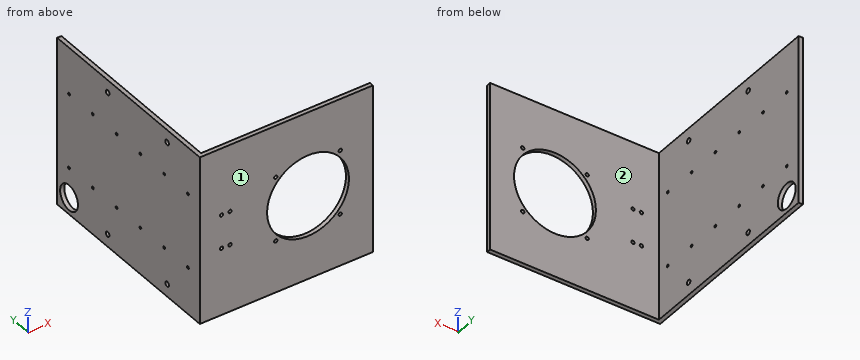
from build123d import *

# Parameters (mm, degrees)
BOSS_EXTRUDE1_DEPTH = 200
CUT_EXTRUDE1_REACH  = 372.473
SKETCH2_R           = 48.5
SKETCH2_R_2         = 2
CUT_EXTRUDE2_REACH  = 372.473
SKETCH3_R           = 2
SKETCH4_R           = 15
CUT_EXTRUDE3_DEPTH  = 10
CUT_EXTRUDE4_REACH  = 372.945
SKETCH5_R           = 3
CUT_EXTRUDE5_REACH  = 372.945
SKETCH6_R           = 1.5


with BuildPart() as part:
    # Sketch1 → Boss-Extrude1 (new body)
    with BuildSketch(Plane.XY):
        Polygon((0, 240), (0, 0), (205, 0), (205, 5), (5, 5), (5, 240), align=None)
    extrude(amount=BOSS_EXTRUDE1_DEPTH)

    # Sketch2 → Cut-Extrude1 (cut, up to next)
    with BuildSketch(Plane(origin=(0, 5, 0), x_dir=(1, 0, 0), z_dir=(0, 1, 0)), mode=Mode.PRIVATE) as cut_extrude1_sk1:
        with Locations(Location((128.16761425, -100, 0), (0, 0, 180))):
            Circle(SKETCH2_R)
    cut_extrude1_tool1 = extrude(cut_extrude1_sk1.sketch, amount=-CUT_EXTRUDE1_REACH, mode=Mode.PRIVATE) & part.part
    # Sketch2 → Cut-Extrude1 (cut, up to next)
    with BuildSketch(Plane(origin=(0, 5, 0), x_dir=(1, 0, 0), z_dir=(0, 1, 0)), mode=Mode.PRIVATE) as cut_extrude1_sk2:
        with Locations(Location((89.98261425, -61.817467672, 0), (0, 0, 180))):
            Circle(SKETCH2_R_2)
    cut_extrude1_tool2 = extrude(cut_extrude1_sk2.sketch, amount=-CUT_EXTRUDE1_REACH, mode=Mode.PRIVATE) & part.part
    # Sketch2 → Cut-Extrude1 (cut, up to next)
    with BuildSketch(Plane(origin=(0, 5, 0), x_dir=(1, 0, 0), z_dir=(0, 1, 0)), mode=Mode.PRIVATE) as cut_extrude1_sk3:
        with Locations(Location((166.35261425, -61.817467672, 0), (0, 0, 180))):
            Circle(SKETCH2_R_2)
    cut_extrude1_tool3 = extrude(cut_extrude1_sk3.sketch, amount=-CUT_EXTRUDE1_REACH, mode=Mode.PRIVATE) & part.part
    # Sketch2 → Cut-Extrude1 (cut, up to next)
    with BuildSketch(Plane(origin=(0, 5, 0), x_dir=(1, 0, 0), z_dir=(0, 1, 0)), mode=Mode.PRIVATE) as cut_extrude1_sk4:
        with Locations(Location((89.98261425, -138.182532328, 0), (0, 0, 180))):
            Circle(SKETCH2_R_2)
    cut_extrude1_tool4 = extrude(cut_extrude1_sk4.sketch, amount=-CUT_EXTRUDE1_REACH, mode=Mode.PRIVATE) & part.part
    # Sketch2 → Cut-Extrude1 (cut, up to next)
    with BuildSketch(Plane(origin=(0, 5, 0), x_dir=(1, 0, 0), z_dir=(0, 1, 0)), mode=Mode.PRIVATE) as cut_extrude1_sk5:
        with Locations(Location((166.35261425, -138.182532328, 0), (0, 0, 180))):
            Circle(SKETCH2_R_2)
    cut_extrude1_tool5 = extrude(cut_extrude1_sk5.sketch, amount=-CUT_EXTRUDE1_REACH, mode=Mode.PRIVATE) & part.part
    add(cut_extrude1_tool1.solids().sort_by_distance((128.167614, 5, 100))[0], mode=Mode.SUBTRACT)
    add(cut_extrude1_tool2.solids().sort_by_distance((89.982614, 5, 61.817468))[0], mode=Mode.SUBTRACT)
    add(cut_extrude1_tool3.solids().sort_by_distance((166.352614, 5, 61.817468))[0], mode=Mode.SUBTRACT)
    add(cut_extrude1_tool4.solids().sort_by_distance((89.982614, 5, 138.182532))[0], mode=Mode.SUBTRACT)
    add(cut_extrude1_tool5.solids().sort_by_distance((166.352614, 5, 138.182532))[0], mode=Mode.SUBTRACT)

    # Sketch3 → Cut-Extrude2 (cut, up to next)
    with BuildSketch(Plane(origin=(0, 5, 0), x_dir=(1, 0, 0), z_dir=(0, 1, 0)), mode=Mode.PRIVATE) as cut_extrude2_sk1:
        with Locations(Location((25.75, -80, 0), (0, 0, 180))):
            Circle(SKETCH3_R)
    cut_extrude2_tool1 = extrude(cut_extrude2_sk1.sketch, amount=-CUT_EXTRUDE2_REACH, mode=Mode.PRIVATE) & part.part
    # Sketch3 → Cut-Extrude2 (cut, up to next)
    with BuildSketch(Plane(origin=(0, 5, 0), x_dir=(1, 0, 0), z_dir=(0, 1, 0)), mode=Mode.PRIVATE) as cut_extrude2_sk2:
        with Locations(Location((25.75, -120, 0), (0, 0, 270))):
            Circle(SKETCH3_R)
    cut_extrude2_tool2 = extrude(cut_extrude2_sk2.sketch, amount=-CUT_EXTRUDE2_REACH, mode=Mode.PRIVATE) & part.part
    # Sketch3 → Cut-Extrude2 (cut, up to next)
    with BuildSketch(Plane(origin=(0, 5, 0), x_dir=(1, 0, 0), z_dir=(0, 1, 0)), mode=Mode.PRIVATE) as cut_extrude2_sk3:
        with Locations(Location((35.75, -120, 0), (0, 0, 180))):
            Circle(SKETCH3_R)
    cut_extrude2_tool3 = extrude(cut_extrude2_sk3.sketch, amount=-CUT_EXTRUDE2_REACH, mode=Mode.PRIVATE) & part.part
    # Sketch3 → Cut-Extrude2 (cut, up to next)
    with BuildSketch(Plane(origin=(0, 5, 0), x_dir=(1, 0, 0), z_dir=(0, 1, 0)), mode=Mode.PRIVATE) as cut_extrude2_sk4:
        with Locations(Location((35.75, -80, 0), (0, 0, 270))):
            Circle(SKETCH3_R)
    cut_extrude2_tool4 = extrude(cut_extrude2_sk4.sketch, amount=-CUT_EXTRUDE2_REACH, mode=Mode.PRIVATE) & part.part
    add(cut_extrude2_tool1.solids().sort_by_distance((25.75, 5, 80))[0], mode=Mode.SUBTRACT)
    add(cut_extrude2_tool2.solids().sort_by_distance((25.75, 5, 120))[0], mode=Mode.SUBTRACT)
    add(cut_extrude2_tool3.solids().sort_by_distance((35.75, 5, 120))[0], mode=Mode.SUBTRACT)
    add(cut_extrude2_tool4.solids().sort_by_distance((35.75, 5, 80))[0], mode=Mode.SUBTRACT)

    # Sketch4 → Cut-Extrude3 (cut)
    with BuildSketch(Plane(origin=(5, 0, 0), x_dir=(0, 0, -1), z_dir=(1, 0, 0))):
        with Locations(Location((-20, 220, 0), (0, 0, 90))):
            Circle(SKETCH4_R)
    extrude(amount=-CUT_EXTRUDE3_DEPTH, mode=Mode.SUBTRACT)

    # Sketch5 → Cut-Extrude4 (cut, up to next)
    with BuildSketch(Plane(origin=(5, 0, 0), x_dir=(0, 0, -1), z_dir=(1, 0, 0)), mode=Mode.PRIVATE) as cut_extrude4_sk1:
        with Locations(Location((-185, 55, 0), (0, 0, 90))):
            Circle(SKETCH5_R)
    cut_extrude4_tool1 = extrude(cut_extrude4_sk1.sketch, amount=-CUT_EXTRUDE4_REACH, mode=Mode.PRIVATE) & part.part
    # Sketch5 → Cut-Extrude4 (cut, up to next)
    with BuildSketch(Plane(origin=(5, 0, 0), x_dir=(0, 0, -1), z_dir=(1, 0, 0)), mode=Mode.PRIVATE) as cut_extrude4_sk2:
        with Locations(Location((-185, 155, 0), (0, 0, 90))):
            Circle(SKETCH5_R)
    cut_extrude4_tool2 = extrude(cut_extrude4_sk2.sketch, amount=-CUT_EXTRUDE4_REACH, mode=Mode.PRIVATE) & part.part
    # Sketch5 → Cut-Extrude4 (cut, up to next)
    with BuildSketch(Plane(origin=(5, 0, 0), x_dir=(0, 0, -1), z_dir=(1, 0, 0)), mode=Mode.PRIVATE) as cut_extrude4_sk3:
        with Locations(Location((-15, 55, 0), (0, 0, 90))):
            Circle(SKETCH5_R)
    cut_extrude4_tool3 = extrude(cut_extrude4_sk3.sketch, amount=-CUT_EXTRUDE4_REACH, mode=Mode.PRIVATE) & part.part
    # Sketch5 → Cut-Extrude4 (cut, up to next)
    with BuildSketch(Plane(origin=(5, 0, 0), x_dir=(0, 0, -1), z_dir=(1, 0, 0)), mode=Mode.PRIVATE) as cut_extrude4_sk4:
        with Locations(Location((-15, 155, 0), (0, 0, 90))):
            Circle(SKETCH5_R)
    cut_extrude4_tool4 = extrude(cut_extrude4_sk4.sketch, amount=-CUT_EXTRUDE4_REACH, mode=Mode.PRIVATE) & part.part
    add(cut_extrude4_tool1.solids().sort_by_distance((5, 55, 185))[0], mode=Mode.SUBTRACT)
    add(cut_extrude4_tool2.solids().sort_by_distance((5, 155, 185))[0], mode=Mode.SUBTRACT)
    add(cut_extrude4_tool3.solids().sort_by_distance((5, 55, 15))[0], mode=Mode.SUBTRACT)
    add(cut_extrude4_tool4.solids().sort_by_distance((5, 155, 15))[0], mode=Mode.SUBTRACT)

    # Sketch6 → Cut-Extrude5 (cut, up to next)
    with BuildSketch(Plane(origin=(5, 0, 0), x_dir=(0, 0, -1), z_dir=(1, 0, 0)), mode=Mode.PRIVATE) as cut_extrude5_sk1:
        with Locations(Location((-144.25, 220, 0), (0, 0, 90))):
            Circle(SKETCH6_R)
    cut_extrude5_tool1 = extrude(cut_extrude5_sk1.sketch, amount=-CUT_EXTRUDE5_REACH, mode=Mode.PRIVATE) & part.part
    # Sketch6 → Cut-Extrude5 (cut, up to next)
    with BuildSketch(Plane(origin=(5, 0, 0), x_dir=(0, 0, -1), z_dir=(1, 0, 0)), mode=Mode.PRIVATE) as cut_extrude5_sk2:
        with Locations(Location((-55.75, 220, 0), (0, 0, 90))):
            Circle(SKETCH6_R)
    cut_extrude5_tool2 = extrude(cut_extrude5_sk2.sketch, amount=-CUT_EXTRUDE5_REACH, mode=Mode.PRIVATE) & part.part
    # Sketch6 → Cut-Extrude5 (cut, up to next)
    with BuildSketch(Plane(origin=(5, 0, 0), x_dir=(0, 0, -1), z_dir=(1, 0, 0)), mode=Mode.PRIVATE) as cut_extrude5_sk3:
        with Locations(Location((-144.25, 180, 0), (0, 0, 90))):
            Circle(SKETCH6_R)
    cut_extrude5_tool3 = extrude(cut_extrude5_sk3.sketch, amount=-CUT_EXTRUDE5_REACH, mode=Mode.PRIVATE) & part.part
    # Sketch6 → Cut-Extrude5 (cut, up to next)
    with BuildSketch(Plane(origin=(5, 0, 0), x_dir=(0, 0, -1), z_dir=(1, 0, 0)), mode=Mode.PRIVATE) as cut_extrude5_sk4:
        with Locations(Location((-55.75, 180, 0), (0, 0, 90))):
            Circle(SKETCH6_R)
    cut_extrude5_tool4 = extrude(cut_extrude5_sk4.sketch, amount=-CUT_EXTRUDE5_REACH, mode=Mode.PRIVATE) & part.part
    # Sketch6 → Cut-Extrude5 (cut, up to next)
    with BuildSketch(Plane(origin=(5, 0, 0), x_dir=(0, 0, -1), z_dir=(1, 0, 0)), mode=Mode.PRIVATE) as cut_extrude5_sk5:
        with Locations(Location((-144.25, 140, 0), (0, 0, 90))):
            Circle(SKETCH6_R)
    cut_extrude5_tool5 = extrude(cut_extrude5_sk5.sketch, amount=-CUT_EXTRUDE5_REACH, mode=Mode.PRIVATE) & part.part
    # Sketch6 → Cut-Extrude5 (cut, up to next)
    with BuildSketch(Plane(origin=(5, 0, 0), x_dir=(0, 0, -1), z_dir=(1, 0, 0)), mode=Mode.PRIVATE) as cut_extrude5_sk6:
        with Locations(Location((-55.75, 140, 0), (0, 0, 90))):
            Circle(SKETCH6_R)
    cut_extrude5_tool6 = extrude(cut_extrude5_sk6.sketch, amount=-CUT_EXTRUDE5_REACH, mode=Mode.PRIVATE) & part.part
    # Sketch6 → Cut-Extrude5 (cut, up to next)
    with BuildSketch(Plane(origin=(5, 0, 0), x_dir=(0, 0, -1), z_dir=(1, 0, 0)), mode=Mode.PRIVATE) as cut_extrude5_sk7:
        with Locations(Location((-144.25, 100, 0), (0, 0, 90))):
            Circle(SKETCH6_R)
    cut_extrude5_tool7 = extrude(cut_extrude5_sk7.sketch, amount=-CUT_EXTRUDE5_REACH, mode=Mode.PRIVATE) & part.part
    # Sketch6 → Cut-Extrude5 (cut, up to next)
    with BuildSketch(Plane(origin=(5, 0, 0), x_dir=(0, 0, -1), z_dir=(1, 0, 0)), mode=Mode.PRIVATE) as cut_extrude5_sk8:
        with Locations(Location((-55.75, 100, 0), (0, 0, 90))):
            Circle(SKETCH6_R)
    cut_extrude5_tool8 = extrude(cut_extrude5_sk8.sketch, amount=-CUT_EXTRUDE5_REACH, mode=Mode.PRIVATE) & part.part
    # Sketch6 → Cut-Extrude5 (cut, up to next)
    with BuildSketch(Plane(origin=(5, 0, 0), x_dir=(0, 0, -1), z_dir=(1, 0, 0)), mode=Mode.PRIVATE) as cut_extrude5_sk9:
        with Locations(Location((-144.25, 60, 0), (0, 0, 90))):
            Circle(SKETCH6_R)
    cut_extrude5_tool9 = extrude(cut_extrude5_sk9.sketch, amount=-CUT_EXTRUDE5_REACH, mode=Mode.PRIVATE) & part.part
    # Sketch6 → Cut-Extrude5 (cut, up to next)
    with BuildSketch(Plane(origin=(5, 0, 0), x_dir=(0, 0, -1), z_dir=(1, 0, 0)), mode=Mode.PRIVATE) as cut_extrude5_sk10:
        with Locations(Location((-55.75, 60, 0), (0, 0, 90))):
            Circle(SKETCH6_R)
    cut_extrude5_tool10 = extrude(cut_extrude5_sk10.sketch, amount=-CUT_EXTRUDE5_REACH, mode=Mode.PRIVATE) & part.part
    # Sketch6 → Cut-Extrude5 (cut, up to next)
    with BuildSketch(Plane(origin=(5, 0, 0), x_dir=(0, 0, -1), z_dir=(1, 0, 0)), mode=Mode.PRIVATE) as cut_extrude5_sk11:
        with Locations(Location((-144.25, 20, 0), (0, 0, 90))):
            Circle(SKETCH6_R)
    cut_extrude5_tool11 = extrude(cut_extrude5_sk11.sketch, amount=-CUT_EXTRUDE5_REACH, mode=Mode.PRIVATE) & part.part
    # Sketch6 → Cut-Extrude5 (cut, up to next)
    with BuildSketch(Plane(origin=(5, 0, 0), x_dir=(0, 0, -1), z_dir=(1, 0, 0)), mode=Mode.PRIVATE) as cut_extrude5_sk12:
        with Locations(Location((-55.75, 20, 0), (0, 0, 90))):
            Circle(SKETCH6_R)
    cut_extrude5_tool12 = extrude(cut_extrude5_sk12.sketch, amount=-CUT_EXTRUDE5_REACH, mode=Mode.PRIVATE) & part.part
    add(cut_extrude5_tool1.solids().sort_by_distance((5, 220, 144.25))[0], mode=Mode.SUBTRACT)
    add(cut_extrude5_tool2.solids().sort_by_distance((5, 220, 55.75))[0], mode=Mode.SUBTRACT)
    add(cut_extrude5_tool3.solids().sort_by_distance((5, 180, 144.25))[0], mode=Mode.SUBTRACT)
    add(cut_extrude5_tool4.solids().sort_by_distance((5, 180, 55.75))[0], mode=Mode.SUBTRACT)
    add(cut_extrude5_tool5.solids().sort_by_distance((5, 140, 144.25))[0], mode=Mode.SUBTRACT)
    add(cut_extrude5_tool6.solids().sort_by_distance((5, 140, 55.75))[0], mode=Mode.SUBTRACT)
    add(cut_extrude5_tool7.solids().sort_by_distance((5, 100, 144.25))[0], mode=Mode.SUBTRACT)
    add(cut_extrude5_tool8.solids().sort_by_distance((5, 100, 55.75))[0], mode=Mode.SUBTRACT)
    add(cut_extrude5_tool9.solids().sort_by_distance((5, 60, 144.25))[0], mode=Mode.SUBTRACT)
    add(cut_extrude5_tool10.solids().sort_by_distance((5, 60, 55.75))[0], mode=Mode.SUBTRACT)
    add(cut_extrude5_tool11.solids().sort_by_distance((5, 20, 144.25))[0], mode=Mode.SUBTRACT)
    add(cut_extrude5_tool12.solids().sort_by_distance((5, 20, 55.75))[0], mode=Mode.SUBTRACT)


solid = part.part
Work out the finished part from the listing and answer in its coordinate system (mm). Face numbers are marked on the shaded views. A direction names the side the tool comes from. Round coordinates to 2 decimals unless told otherwise and drop trailing zeros. Write each loop counter-clockwise with the first axis right and the second up, starting at its lowest first coordinate (ties: lowest second). Pieces come first, ordered by that corner, then holes. Notation, with made-up numbers: (13, 73.25) -> (25, 73.25) arc R28 cw to (25, 105.25) -> close; hole circle Ø7 at (-26, -33.5). An arc over 180 degrees is marked (long way). Answer as CSV lines item,"result". Start each with the question number.
(1) Find the intervals of material crossed by probe 1 along Z at (x, y) = (1.85, 140); probe 2 along Z at (x, y) = (2.45, 155); probe 3 along X at (y, z) = (85, 183), in increasing order.
(2) The part is cut by section B-B, the plane x = 124.5. Give the vertices of the cut face in (y, z).
(3) A tool of negligible diameter and unlimited length cuts with its end or side. For the marked faces 1 and 2, from which of +Z, -Z, +X, -X, +Y, -Y can it reach the whole face along a straight path? Write none if from no direction.
(4) The part is cut by section D-D, the plane x = 99. Give the vertices of the cut face in (y, z).
(5) The part is cut by section C-C, the plane z = 174.5. Give the vertices of the cut face in (x, y).
(6) The part is cut by section A-A, the plane z = 100. Give the vertices of the cut face in (x, y).
(7) Each of these flat-tipped pins is pushed along its axis until it touches: pin 1 (2.5 mm diameter, centred on y = 180, z = 144.25, fed in from +X); pin 2 (5 mm diameter, centred on x = 115, z = 33, fed in from +Y); pin 3 (2 mm diameter, centred on x = 177, z = 75, fed in from -Y); pin 4 (3.5 mm diameter, centred on y = 140, z = 55.75, fed in from +X). Where does it stop, or does it pass through?
Output values:
1,probe 1,"z = 0 to 54.25, 57.25 to 142.75, 145.75 to 200"
1,probe 2,"z = 0 to 12, 18 to 182, 188 to 200"
1,probe 3,"x = 0 to 5"
2,outline,"(0, 0) -> (5, 0) -> (5, 51.64) -> (0, 51.64) -> close; (0, 148.36) -> (5, 148.36) -> (5, 200) -> (0, 200) -> close"
3,face 1,"+Z, -Z, +X, -X, -Y"
3,face 2,"+Z, -Z, +X, +Y"
4,outline,"(0, 0) -> (5, 0) -> (5, 61.25) -> (0, 61.25) -> close; (0, 138.75) -> (5, 138.75) -> (5, 200) -> (0, 200) -> close"
5,outline,"(0, 0) -> (205, 0) -> (205, 5) -> (5, 5) -> (5, 240) -> (0, 240) -> close"
6,outline,"(0, 0) -> (79.67, 0) -> (79.67, 5) -> (5, 5) -> (5, 240) -> (0, 240) -> close; (176.67, 0) -> (205, 0) -> (205, 5) -> (176.67, 5) -> close"
7,pin 1,"passes through"
7,pin 2,"stops at y = 5"
7,pin 3,"stops at y = 0"
7,pin 4,"stops at x = 5"
